CAD build for the part. Positions are in the model's coordinates, mm. A direction names the side the tool comes from. Round coordinates to 2 decimals unless told otherwise and drop trailing zeros. Loops run counter-clockwise (first coordinate to the right, second up) from the corner with the lowest first, then second, coordinate; pieces in that order, holes last. Notation, with made-up numbers: M 82.25,71.25 L 130.25,71.25 A14 ccw 130.25,94.25 Z; hole C -10.5,10.25 d5. An arc over 180 degrees is marked long. Use a Markdown table: item, result. Add a question column.
(1) Band-saw the part on A-A, the plane z = 0. Write the cut outline in (x, y).
(2) Flat gauge pins, fed straight in: P1, Ø1.5, axis at y = 43, z = 5, coming from the +X side; P2, Ø5, axis at x = 4.5, y = 54.5, coming from the -Z side; P3, Ø3, axis at y = 38.5, z = -5, coming from the -X side. Where does each tip first touch, or does it go through?
(3) Two-plate mould, pull along X, no slides. Class faces 4 (the face through (-3, -6, 0)), 5 (the face through (-1.32, -4.13, -2.24)), 6 (the face through (-4.88, 32.66, -1.08)): released by +X, released by -X, zero draft, split by the parting line, or undercut.
(4) Band-saw the part on C-C, the plane z = 6.25. Write the cut outline in (x, y), and give its area (3 significant figures).
(5) Band-saw the part on B-B, the plane y = 24.5. Write the cut outline in (x, z).
(6) Which spindle directions (+Z, -Z, +X, -X, +Y, -Y) get a long thin tool onto all of the face, cutting with end or side? Do faces 1 (the face through (0, 67, 0)), 2 (the face through (5, 0, 2)), 3 (the face through (2.6, -4, 0)). Say none if no direction does.
(7) Wall check: L1, parallel to Y at x = -1.75, z = -1.5; L2, parallel to Y at x = 3.25, z = -4; L3, parallel to X at y = 3.5, z = -4. Give the ranges that are in metal, low to high.
from build123d import *

# Parameters (mm, degrees)
SKETCH1_R           = 5
BOSS_EXTRUDE1_DEPTH = 67
CHAMFER1_SIZE       = 0.75
SKETCH2_R           = 7
BOSS_EXTRUDE2_DEPTH = 6
CUT_EXTRUDE1_DEPTH  = 3.8


with BuildPart() as part:
    # Sketch1 → Boss-Extrude1 (new body)
    with BuildSketch(Plane(origin=(0, 0, 0), x_dir=(1, 0, 0), z_dir=(0, 1, 0))):
        with Locations(Location((0, 0, 0), (0, 0, 270))):
            Circle(SKETCH1_R)
    extrude(amount=BOSS_EXTRUDE1_DEPTH)

    # Chamfer1
    chamfer1_edges = [part.edges().sort_by_distance(p)[0] for p in [
        (0, 67, -5),
    ]]
    chamfer(chamfer1_edges, length=CHAMFER1_SIZE)

    # Sketch2 → Boss-Extrude2 (add)
    with BuildSketch(Plane.XZ):
        with Locations(Location((0, 0, 0), (0, 0, 270))):
            Circle(SKETCH2_R)
    extrude(amount=BOSS_EXTRUDE2_DEPTH)

    # Sketch3 → Cut-Extrude1 (cut)
    with BuildSketch(Plane.XZ.offset(6)):
        Polygon((0, 3.0022214), (-2.6, 1.5011107), (-2.6, -1.5011107), (0, -3.0022214), (2.6, -1.5011107), (2.6, 1.5011107), align=None)
    extrude(amount=-CUT_EXTRUDE1_DEPTH, mode=Mode.SUBTRACT)


solid = part.part
Return value:
| question | item | result |
|---|---|---|
| 1 | outline | M -7,-6 L -2.6,-6 L -2.6,-2.2 L 2.6,-2.2 L 2.6,-6 L 7,-6 L 7,0 L 5,0 L 5,66.25 L 4.25,67 L -4.25,67 L -5,66.25 L -5,0 L -7,0 Z |
| 2 | P1 | x = 2.63 |
| 2 | P2 | z = -4.58 |
| 2 | P3 | x = -3.57 |
| 3 | face 4 | zero draft |
| 3 | face 5 | undercut |
| 3 | face 6 | split by the parting line |
| 4 | outline | M -3.15,-6 L 3.15,-6 L 3.15,0 L -3.15,0 Z |
| 4 | area | 37.8 mm^2 |
| 5 | outline | C 0,0 d10 |
| 6 | face 1 | +Z, -Z, +X, -X, +Y |
| 6 | face 2 | +Y |
| 6 | face 3 | -Y |
| 7 | L1 | -2.2 to 67 |
| 7 | L2 | -6 to 0 |
| 7 | L3 | -3 to 3 |
